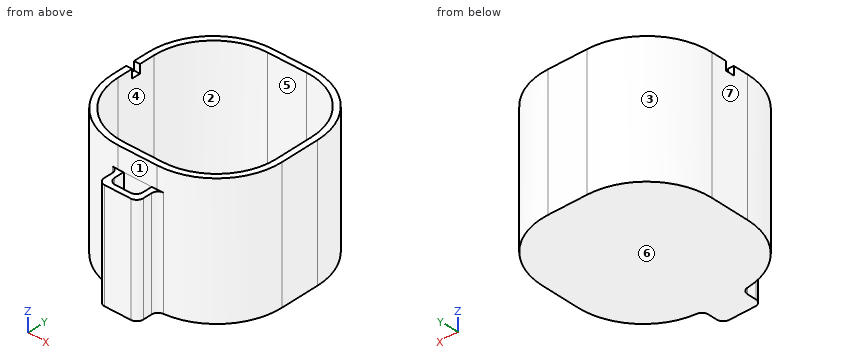
from build123d import *

# Parameters (mm, degrees)
F0_W      = 78
F0_H      = 78
F1_DEPTH  = 60
F2_R      = 30
F4_T      = -2.7
F3_W      = 18
F3_H      = 10
F5_DEPTH  = 25
F6_DEPTH  = 50
F7_T      = -2.5
F8_R      = 5.5856812821
F9_DEPTH  = 25
F10_R     = 3
F11_W     = 2.7
F11_H     = 4
F12_DEPTH = 4


# Not quite as in the source:
# - a shell that OpenCascade refuses in one call is made with other operations: the cavity is built on its own and cut out


with BuildPart() as f1:
    # F0 (on Top) → F1 (new body)
    with BuildSketch(Plane.XY):
        Rectangle(F0_W, F0_H)
    extrude(amount=F1_DEPTH)

    # F2
    f2_edges = [f1.edges().sort_by_distance(p)[0] for p in [
        (-39, -39, 30),
        (39, -39, 30),
        (39, 39, 30),
        (-39, 39, 30),
    ]]
    fillet(f2_edges, radius=F2_R)

    # F4
    f4_openings = [f1.faces().sort_by_distance(p)[0] for p in [
        (0, 0, 60),
    ]]
    offset(amount=F4_T, openings=f4_openings)

    # F3 (on Top) → F5 (cut)
    with BuildSketch(Plane.XY):
        with Locations((0, -44)):
            Rectangle(F3_W, F3_H)
    extrude(amount=-F5_DEPTH, mode=Mode.SUBTRACT)

    # F3 (on Top) → F6 (join)
    with BuildSketch(Plane.XY):
        with Locations((0, -44)):
            Rectangle(F3_W, F3_H)
    extrude(amount=F6_DEPTH)

    # F7: a shell. OpenCascade refuses it in one call, so the cavity is built on its own and cut out:
    # the body offset inwards by the wall thickness, plus a prism from it out through each open face.
    f7_core = offset(f1.part, amount=F7_T, kind=Kind.INTERSECTION, mode=Mode.PRIVATE)
    f7_exits = [f7_core.faces().sort_by_distance(p)[0] for p in [
        (0, -42.65, 47.5),
    ]]
    add(f7_core, mode=Mode.SUBTRACT)
    extrude(f7_exits, amount=-F7_T, mode=Mode.SUBTRACT)

    # F8 (on face) → F9 (cut)
    with BuildSketch(Plane.XZ.offset(39)):
        with Locations((0, 10.1356906816)):
            Circle(F8_R)
    extrude(amount=-F9_DEPTH, mode=Mode.SUBTRACT)

    # F10
    f10_edges = [f1.edges().sort_by_distance(p)[0] for p in [
        (-9, -49, 25),
        (9, -49, 25),
        (-6.5, -46.5, 26.25),
        (6.5, -46.5, 26.25),
        (-9, -39, 25),
        (-9, -39, 55),
        (9, -39, 25),
        (9, -39, 55),
    ]]
    fillet(f10_edges, radius=F10_R)

    # F11 (on face) → F12 (cut)
    with BuildSketch(Plane.XY.offset(60)):
        with Locations((-37.65, 0)):
            Rectangle(F11_W, F11_H)
    extrude(amount=-F12_DEPTH, mode=Mode.SUBTRACT)


solid = f1.part
The model under review builds one solid part; all positions refer to its coordinate system, in mm. Face numbers are marked on the shaded views. A direction names the side the tool comes from. Give positions to 0.01 mm unless a question says otherwise; leave off trailing zeros. Order: outer loops, then holes, each group sorted by start corner. A loop starts at its lowest first (then second) coordinate and runs counter-clockwise, first axis right, second up. Notation, with made-up numbers: M 82,84.5 L 126,84.5 A28 cw 126,105.5 Z; hole C 70.5,-3.75 d4. An arc over 180 degrees is marked long. Use one line per item in the form item = value. Start each with the question number.
Item 1: Insertion check: pin 1 Ø3 at (x, z) = (-3, 53) entering from -Y; pin 2 Ø4 at (x, y) = (3, -42.5) entering from +Z; pin 3 Ø12 at (x, y) = (6, 4.5) entering from +Z. Each pin has a flat end and moves straight along its axis. Give the tip position at first contact, or say it passes through.
Item 2: The part is to be moulded in two halves that separate along X. For the marked faces 4, 5, 6 and 7, say which applies: pulls with the +X half, pulls with the -X half, needs draft (parallel to the pull), parting line crosses it, or undercut.
Item 3: For the marked faces 1, 2 and 3, list the 3-axis set-ups (+Z, -Z, +X, -X, +Y, -Y) from which the entire face can be reached by the end or side of a thin tool; tool diameter is ignored.
Item 4: We need section C-C on y = -11. Give the boundary of the cut face in (x, z).
Item 5: To check wall thickness, follow line 1 along Y through (x, z) = (-3.5, 43); line 2 along X through (y, z) = (1.5, 18.5); line 3 along Z through (x, y) = (0, -37.8). State the ranges of each line that lie inside material, in increasing order. Write a range as from..to.
Item 6: We need section B-B on z = 41.5. Give the boundary of the cut face in (x, y).
Item 7: We need section D-D on x = 34. Give the boundary of the cut face in (y, z), plus the area to 3 significant figures.
Item 8: We need section A-A on x = 0. Give the boundary of the cut face in (y, z), plus the area to 3 significant figures.
Completed:
q1.pin_1 = -39
q1.pin_2 = 2.5
q1.pin_3 = 2.7
q2.face_4 = undercut
q2.face_5 = undercut
q2.face_6 = needs draft
q2.face_7 = pulls with the -X half
q3.face_1 = +Z, +X, -X, -Y
q3.face_2 = +Z
q3.face_3 = +Z, -Z, -X, +Y
q4.outline = M -38.93,0 L 38.93,0 L 38.93,60 L 36.23,60 L 36.23,2.7 L -36.23,2.7 L -36.23,60 L -38.93,60 Z
q5.line_1 = -49..-46.5, -38.8..-36.3, 36.3..39
q5.line_2 = -39..-36.3, 36.3..39
q5.line_3 = 0..4.55, 15.72..60
q6.outline = M -39,-9 A30 ccw -11.73,-38.88 A3 cw -9,-41.86 L -9,-46 A3 ccw -6,-49 L 6,-49 A3 ccw 9,-46 L 9,-41.86 A3 cw 11.73,-38.88 A30 ccw 39,-9 L 39,9 A30 ccw 9,39 L -9,39 A30 ccw -39,9 Z; hole M -36.3,-9 A27.3 ccw -9,-36.3 L 9,-36.3 A27.3 ccw 36.3,-9 L 36.3,9 A27.3 ccw 9,36.3 L -9,36.3 A27.3 ccw -36.3,9 Z; hole M -6.5,-43.5 A3 ccw -3.5,-46.5 L 3.5,-46.5 A3 ccw 6.5,-43.5 L 6.5,-38.8 L -6.5,-38.8 Z
q7.outline = M -25.58,0 L 25.58,0 L 25.58,60 L 19.97,60 L 19.97,2.7 L -19.97,2.7 L -19.97,60 L -25.58,60 Z
q7.area = 782 mm²
q8.outline = M -49,0 L 39,0 L 39,60 L 36.3,60 L 36.3,2.7 L -36.3,2.7 L -36.3,4.55 L -38.8,4.55 L -38.8,2.5 L -46.5,2.5 L -46.5,50 L -49,50 Z; M -39,50 L -38.8,50 L -38.8,15.72 L -36.3,15.72 L -36.3,60 L -39,60 Z
q8.area = 626 mm²
